Answer from the drawing. Dimensions are ordinates in mm from the lowest x, y and z of the part. A direction names the side the tool comes from. Round coordinates to 2 decimals unless told otherwise and drop trailing zeros. Write each loop counter-clockwise with the first axis right and the second up, starting at its lowest first coordinate (ties: lowest second). Pieces come first, ordered by that corner, then holes. Notation, with made-up numbers: (-18.5, -17.5) -> (14.5, -17.5) arc R11 cw to (14.5, 2.5) -> close; hole circle Ø2 at (-24.5, 70.5). An arc over 180 degrees is marked (long way). Return JSON: item names as keys, results as strings. Group by question number.
(1) For the marked faces 1, 2 and 3, determine the directions among +Z, -Z, +X, -X, +Y, -Y from which every point of the face is accessible in a straight line to the end or side of a thin tool.
(2) A cutting plane is placed at A-A on z = 25.4. Give the vertices of the cut face in (x, y).
(3) The mould has two halves that part along Z. Classify the marked faces 4 and 5: released by +Z, released by -Z, zero draft, split by the parting line, or undercut.
(4) Given pin 1 (1 mm diameter, centred on x = 127.5, y = 17.5, fed in from -Z); pin 2 (2 mm diameter, centred on x = 209, y = 6, fed in from +Z); pin 3 (4 mm diameter, centred on y = 7.5, z = 10, fed in from +X), each flat-ended and moving along its own axis, determine where each tip first touches the part or whether it passes through.
(5) A cutting plane is placed at C-C on x = 87.5. Give the vertices of the cut face in (y, z), then the cut area to 3 significant figures.
(6) A cutting plane is placed at D-D on y = 41.5. Give the vertices of the cut face in (x, z), then the cut area to 3 significant figures.
(7) Straight lines are drawn through the part: line 1 (X direction, y = 11, z = 7); line 2 (Y direction, x = 287.5, z = 23.5); line 3 (Y direction, x = 255, z = 30). For each, find the intervals that lie inside material, in ascending order.
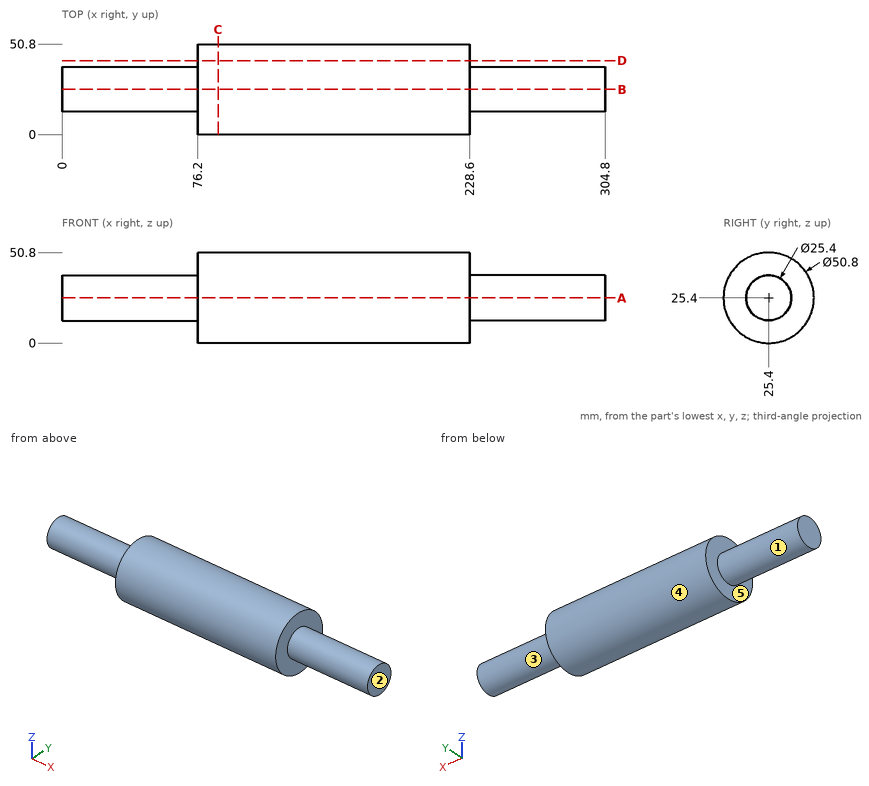
Checks:
{
 "1": {"face 1": "-X", "face 2": "+Z, -Z, +X, +Y, -Y", "face 3": "+X"},
 "2": {"outline": "(0, 12.7) -> (76.2, 12.7) -> (76.2, 0) -> (228.6, 0) -> (228.6, 12.7) -> (304.8, 12.7) -> (304.8, 38.1) -> (228.6, 38.1) -> (228.6, 50.8) -> (76.2, 50.8) -> (76.2, 38.1) -> (0, 38.1) -> close"},
 "3": {"face 4": "split by the parting line", "face 5": "zero draft"},
 "4": {"pin 1": "stops at z = 1.1", "pin 2": "stops at z = 42.91", "pin 3": "stops at x = 228.6"},
 "5": {"outline": "circle Ø50.8 at (25.4, 25.4)", "area": "2,030 mm^2"},
 "6": {"outline": "(76.2, 5.75) -> (228.6, 5.75) -> (228.6, 45.05) -> (76.2, 45.05) -> close", "area": "5,990 mm^2"},
 "7": {"line 1": "x = 76.2 to 228.6", "line 2": "y = 12.84 to 37.96", "line 3": "y = 13.56 to 37.24"}
}
